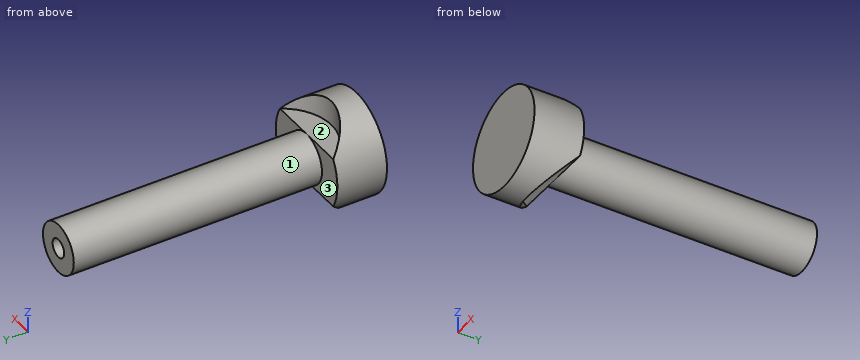
```python
from build123d import *

# Parameters (mm, degrees)
SKETCH1_R           = 6.35
BOSS_EXTRUDE1_DEPTH = 63.5
SKETCH5_R           = 12.7
BOSS_EXTRUDE2_DEPTH = 12.7
SKETCH10_R          = 12.7
CUT_EXTRUDE5_DEPTH  = 68.501425911
SKETCH12_R          = 12.7
CUT_EXTRUDE6_DEPTH  = 68.501425911
SKETCH13_R          = 2.38125
CUT_EXTRUDE7_DEPTH  = 50.8


with BuildPart() as part:
    # Sketch1 → Boss-Extrude1 (new body)
    with BuildSketch(Plane(origin=(0, 0, 0), x_dir=(1, 0, 0), z_dir=(0, 1, 0))):
        with Locations(Location((0, 0, 0), (0, 0, 270))):
            Circle(SKETCH1_R)
    extrude(amount=BOSS_EXTRUDE1_DEPTH)

    # Sketch5 → Boss-Extrude2 (add)
    with BuildSketch(Plane.XZ):
        with Locations(Location((0, 0, 0), (0, 0, 270))):
            Circle(SKETCH5_R)
    extrude(amount=BOSS_EXTRUDE2_DEPTH)

    # Sketch10 → Cut-Extrude5 (cut, through all)
    with BuildSketch(Plane.XY.offset(6.35)):
        with Locations((0, 6.35)):
            Circle(SKETCH10_R)
    extrude(amount=CUT_EXTRUDE5_DEPTH, mode=Mode.SUBTRACT)

    # Sketch12 → Cut-Extrude6 (cut, through all)
    with BuildSketch(Plane(origin=(0, 0, -6.35), x_dir=(-1, 0, 0), z_dir=(0, 0, -1))):
        with Locations((0, 6.35)):
            Circle(SKETCH12_R)
    extrude(amount=CUT_EXTRUDE6_DEPTH, mode=Mode.SUBTRACT)

    # Sketch13 → Cut-Extrude7 (cut)
    with BuildSketch(Plane(origin=(0, 63.5, 0), x_dir=(1, 0, 0), z_dir=(0, 1, 0))):
        with Locations(Location((0, 0, 0), (0, 0, 270))):
            Circle(SKETCH13_R)
    extrude(amount=-CUT_EXTRUDE7_DEPTH, mode=Mode.SUBTRACT)


solid = part.part
```
Source: CAD feature listing. Evaluate the final solid. Frame: model axes, mm. Face numbers are marked on the shaded views. A direction names the side the tool comes from. Give positions to 0.01 mm unless a question says otherwise; leave off trailing zeros. Write each loop counter-clockwise with the first axis right and the second up, starting at its lowest first coordinate (ties: lowest second). Pieces come first, ordered by that corner, then holes. Notation, with made-up numbers: (30.25, -6.75) - (46.25, -6.75) arc R23 cw to (46.25, 32.25) - close; hole circle Ø3 at (-21.5, 39). An arc over 180 degrees is marked (long way). One line per item, written item: value. Start each with the question number.
Q1. First-contact query: pin 1 Ø7 at (x, y) = (-1.5, -2) entering from +Z; pin 2 Ø5 at (y, z) = (40, 10) entering from -X; pin 3 Ø5 at (x, y) = (-2.5, -4.5) entering from -Z; pin 4 Ø8 at (x, y) = (-8, 8.5) entering from +Z. Flat tips, straight axial feed; report the tip coordinate or a pass-through.
Q2. Material intervals for probe 1 along X at (y, z) = (49.5, 0); probe 2 along Y at (x, z) = (11.25, 5.75); probe 3 along X at (y, z) = (39, 1.25), sorted ascending. Write a range as from..to.
Q3. Section query A-A, the plane z = 0. Return the cut outline in (x, y), then the cut area to 3 significant figures.
Q4. Section query B-B, the plane y = 32. Return the cut outline in (x, z), then the cut area to 3 significant figures.
Q5. Section query C-C, the plane x = -1. Return the cut outline in (y, z).
Q6. Set-up query: the marked faces 1, 2 and 3. Return all of +Z, -Z, +X, -X, +Y, -Y with unobstructed straight access to the full face (end or side cutting, diameter ignored); none if empty.
Q7. Section query D-D, the plane y = 11.5. Return the cut outline in (x, z), then the cut area to 3 significant figures.
Answer:
1. pin 1: stops at z = 6.35
1. pin 2: passes through
1. pin 3: stops at z = -12.68
1. pin 4: stops at z = 4.93
2. probe 1: x = -6.35..-2.38, 2.38..6.35
2. probe 2: y = -12.7..0
2. probe 3: x = -6.23..-2.03, 2.03..6.23
3. outline: (-12.7, -12.7) - (12.7, -12.7) - (12.7, 0) - (6.35, 0) - (6.35, 63.5) - (2.38, 63.5) - (2.38, 12.7) - (-2.38, 12.7) - (-2.38, 63.5) - (-6.35, 63.5) - (-6.35, 0) - (-12.7, 0) - close
3. area: 887 mm2
4. outline: circle Ø12.7 at (0, 0); hole circle Ø4.76 at (0, 0)
4. area: 109 mm2
5. outline: (-12.7, -12.66) - (-6.31, -12.66) - (-6.31, -6.35) - (0, -6.35) - (0, -6.27) - (63.5, -6.27) - (63.5, -2.16) - (12.7, -2.16) - (12.7, 2.16) - (63.5, 2.16) - (63.5, 6.27) - (0, 6.27) - (0, 6.35) - (-6.31, 6.35) - (-6.31, 12.66) - (-12.7, 12.66) - close
6. face 1: +Y
6. face 2: +Z, +Y
6. face 3: -X, +Y
7. outline: circle Ø12.7 at (0, 0)
7. area: 127 mm2
